from build123d import *

# Parameters (mm, degrees)
BOSS_EXTRU_1_DEPTH      = 90
ESQUISSE2_W             = 140
ESQUISSE2_H             = 22
BOSS_EXTRU_2_DEPTH      = 10
ESQUISSE3_R             = 1.7
BOSS_EXTRU_3_DEPTH      = 140
ESQUISSE4_W             = 8
ESQUISSE4_H             = 15.226360619
ESQUISSE4_H_2           = 8
ESQUISSE4_H_3           = 3
ESQUISSE4_W_2           = 96
ENL_V_MAT_EXTRU_1_DEPTH = 10
ESQUISSE6_R             = 2.25
ENL_V_MAT_EXTRU_2_DEPTH = 10
CHANFREIN1_SIZE         = 0.5
CONG_4_R                = 5
CONG_1_R                = 1
ENL_V_MAT_EXTRU_4_DEPTH = 153.159710088


with BuildPart() as part:
    # Esquisse1 → Boss.-Extru.1 (new body)
    with BuildSketch(Plane(origin=(0, 0, 0), x_dir=(1, 0, 0), z_dir=(0, 1, 0))):
        with BuildLine():
            Line((-70, -6.538554455), (-70, -11.538554455))
            Line((-70, -11.538554455), (70, -11.538554455))
            Line((70, -11.538554455), (70, -6.538554455))
            ThreePointArc((70, -6.538554455), (73.525998754, 0.746669281), (71, 8.436043923))
            Line((71, 8.436043923), (80.865168939, 8.436043923))
            ThreePointArc((80.865168939, 8.436043923), (80.548331098, -6.276854674), (70, -16.538554455))
            Line((70, -16.538554455), (-70, -16.538554455))
            ThreePointArc((-70, -16.538554455), (-80.548331098, -6.276854674), (-80.865168939, 8.436043923))
            Line((-80.865168939, 8.436043923), (-71, 8.436043923))
            ThreePointArc((-71, 8.436043923), (-73.525998754, 0.746669281), (-70, -6.538554455))
        make_face()
    extrude(amount=BOSS_EXTRU_1_DEPTH)

    # Esquisse2 → Boss.-Extru.2 (add)
    with BuildSketch(Plane(origin=(0, 71, 0), x_dir=(-1, 0, 0), z_dir=(0, -1, 0))):
        with Locations((0, -27.538554455)):
            Rectangle(ESQUISSE2_W, ESQUISSE2_H)
    extrude(amount=-BOSS_EXTRU_2_DEPTH)

    # Esquisse3 → Boss.-Extru.3 (add)
    with BuildSketch(Plane.ZY.offset(70)):
        with BuildLine():
            Line((38.538554455, 71), (46.538554455, 71))
            ThreePointArc((46.538554455, 71), (51.538554455, 76), (46.538554455, 81))
            Line((46.538554455, 81), (38.538554455, 81))
            Line((38.538554455, 81), (38.538554455, 71))
        make_face()
        with Locations((46.538554455, 76)):
            Circle(ESQUISSE3_R, mode=Mode.SUBTRACT)
    extrude(amount=-BOSS_EXTRU_3_DEPTH)

    # Esquisse4 → Enlèv. mat.-Extru.1 (cut)
    with BuildSketch(Plane(origin=(0, 81, 0), x_dir=(1, 0, 0), z_dir=(0, 1, 0))):
        with Locations((-59, -54.151734765)):
            Rectangle(ESQUISSE4_W, ESQUISSE4_H)
        with Locations((-59, -42.538554455)):
            Rectangle(ESQUISSE4_W, ESQUISSE4_H_2)
        with Locations((-59, -37.038554455)):
            Rectangle(ESQUISSE4_W, ESQUISSE4_H_3)
        with Locations((0, -42.538554455)):
            Rectangle(ESQUISSE4_W_2, ESQUISSE4_H_2)
        with Locations((0, -54.151734765)):
            Rectangle(ESQUISSE4_W_2, ESQUISSE4_H)
        with Locations((59, -54.151734765)):
            Rectangle(ESQUISSE4_W, ESQUISSE4_H)
        with Locations((59, -42.538554455)):
            Rectangle(ESQUISSE4_W, ESQUISSE4_H_2)
        with Locations((59, -37.038554455)):
            Rectangle(ESQUISSE4_W, ESQUISSE4_H_3)
    extrude(amount=-ENL_V_MAT_EXTRU_1_DEPTH, mode=Mode.SUBTRACT)

    # Esquisse6 → Enlèv. mat.-Extru.2 (cut)
    with BuildSketch(Plane.ZY.offset(70)):
        with Locations((46.538554455, 76)):
            Circle(ESQUISSE6_R)
    enl_v_mat_extru_2 = extrude(amount=-ENL_V_MAT_EXTRU_2_DEPTH, mode=Mode.SUBTRACT)

    # Symétrie1: Enlèv. mat.-Extru.2 across plane
    add(enl_v_mat_extru_2.mirror(Plane(origin=(0, 0, 0), x_dir=(0, 0, 1), z_dir=(1, 0, 0))), mode=Mode.SUBTRACT)

    # Chanfrein1
    chanfrein1_edges = [part.edges().sort_by_distance(p)[0] for p in [
        (-70, 76, 44.288554455),
        (70, 76, 44.288554455),
    ]]
    chamfer(chanfrein1_edges, length=CHANFREIN1_SIZE)

    # Congé4
    cong_4_edges = [part.edges().sort_by_distance(p)[0] for p in [
        (48, 76, 38.538554455),
        (-48, 76, 38.538554455),
    ]]
    fillet(cong_4_edges, radius=CONG_4_R)

    # Congé1
    cong_1_edges = [part.edges().sort_by_distance(p)[0] for p in [
        (59, 71, 35.538554455),
        (63, 71, 41.038554455),
        (55, 81, 41.038554455),
        (63, 81, 41.038554455),
        (63, 76, 51.538554455),
        (55, 76, 51.538554455),
        (55, 71, 41.038554455),
        (59, 81, 35.538554455),
        (0, 81, 38.538554455),
        (0, 71, 38.538554455),
        (48, 81, 45.038554455),
        (48, 71, 45.038554455),
        (-48, 71, 45.038554455),
        (-48, 81, 45.038554455),
        (46.535533906, 81, 40.003020549),
        (46.535533906, 71, 40.003020549),
        (-46.535533906, 81, 40.003020549),
        (-46.535533906, 71, 40.003020549),
        (70, 81, 31.538554455),
        (-70, 81, 31.538554455),
        (70, 71, 31.538554455),
        (-70, 71, 31.538554455),
        (70, 76, 51.538554455),
        (-70, 76, 51.538554455),
        (-59, 71, 35.538554455),
        (-55, 71, 41.038554455),
        (-63, 81, 41.038554455),
        (-55, 81, 41.038554455),
        (-55, 76, 51.538554455),
        (-63, 76, 51.538554455),
        (-63, 71, 41.038554455),
        (-59, 81, 35.538554455),
        (48, 76, 51.538554455),
        (-48, 76, 51.538554455),
    ]]
    fillet(cong_1_edges, radius=CONG_1_R)

    # Esquisse8 → Enlèv. mat.-Extru.4 (cut, through all)
    with BuildSketch(Plane.ZY.offset(70)):
        Polygon((45.038554455, 81), (41.788554455, 79.5), (38.538554455, 81), align=None)
    extrude(amount=-ENL_V_MAT_EXTRU_4_DEPTH, mode=Mode.SUBTRACT)


solid = part.part
Read the model definition and answer for the solid it produces. Units are mm, in the model's axes. A direction names the side the tool comes from. Round coordinates to 2 decimals unless told otherwise and drop trailing zeros. Loops run counter-clockwise (first coordinate to the right, second up) from the corner with the lowest first, then second, coordinate; pieces in that order, holes last.
Q1. Determine the mould class of faces 5 (the face through (1, 35, 16.539)), 6 (the face through (63, 76, 41)), 7 (the face through (-66.549, 80.24, 40.186)) for opening direction Z: released by +Z, released by -Z, zero draft, split by the parting line, or undercut.
Q2. Each of these flat-tipped pins is pushed along its axis until it touches: pin 1 (2.5 mm diameter, centred on x = 59, y = 77.5, fed in from +Z); pin 2 (2 mm diameter, centred on x = -10, y = 24.5, fed in from -Z); pin 3 (5.5 mm diameter, centred on y = 78, z = 48, fed in from +X). Where does it stop, or does it pass through?
Q3. Section B-B on y = 32.5 is taken. Write down the section's boundary in (x, z), and give its area (3 significant figures).
Q4. Section C-C on x = -28 is taken. Write down the section's boundary in (y, z).
Q5. Section D-D on y = 76 is taken. Give the number of separate pieces and of enclosed holes in the cut face, and give its area (3 significant figures).
Q6. Which of the six approach directions +Z, -Z, +X, -X, +Y, -Y give full straight-line access (tool end or side, diameter ignored) to faces 1 (the face through (66.451, 80.24, 40.186)), 2 (the face through (-66.296, 73.804, 46.051)), 3 (the face through (-70, 76, 30)), 4 (the face through (-59, 76, 35.539))?
Q7. Section A-A on x = -51.5 is taken. Write down the section's boundary in (y, z), and give its area (3 significant figures).
Q8. Consider probe 1 along X at (y, z) = (19.5, -1.5); probe 2 along Z at (x, y) = (49.75, 76); probe 3 along X at (y, z) = (79.5, 17). Determine where each line is inside the solid, lowest interval first.
Output:
1. face 5: released by +Z
1. face 6: zero draft
1. face 7: undercut
2. pin 1: stops at z = 35.54
2. pin 2: stops at z = 11.54
2. pin 3: stops at x = 70
3. outline: (-80.87, -8.44) - (-71, -8.44) arc R10.8 cw to (-70, 6.54) - (-70, 11.54) - (70, 11.54) - (70, 6.54) arc R10.8 cw to (71, -8.44) - (80.87, -8.44) arc R19.41 ccw to (70, 16.54) - (-70, 16.54) arc R19.41 ccw to start
3. area: 1,100 mm2
4. outline: (0, 11.54) - (90, 11.54) - (90, 16.54) - (81, 16.54) - (81, 37.54) arc R1 ccw to (80, 38.54) - (72, 38.54) arc R1 ccw to (71, 37.54) - (71, 16.54) - (0, 16.54) - close
5. separate pieces: 5
5. enclosed holes: 0
5. area: 4,400 mm2
6. face 1: +X, -X, +Y
6. face 2: -X
6. face 3: +Z, -X, +Y, -Y
6. face 4: +Z, +Y, -Y
7. outline: (0, 11.54) - (90, 11.54) - (90, 16.54) - (81, 16.54) - (81, 38.54) - (79.5, 41.79) - (81, 45.04) - (81, 46.54) arc R5 ccw to (71, 46.54) - (71, 16.54) - (0, 16.54) - close; hole circle Ø3.4 at (76, 46.54)
7. area: 775 mm2
8. probe 1: x = -82.16 to -73.55, 73.55 to 82.16
8. probe 2: z = 11.54 to 44.84, 48.24 to 51.54
8. probe 3: x = -70 to 70
